Here's the drawing with two shaded views (mm, measured from the low corner). I have some questions. A direction names the side the tool comes from. Coordinates: 2 decimals unless noted, no trailing zeros. Loops run counter-clockwise (first coordinate to the right, second up) from the corner with the lowest first, then second, coordinate; pieces in that order, holes last. Notation, with made-up numbers: M 60,-10 L 84,-10 A33 cw 84,26 Z; hole C 78.25,58.5 d4. An arc over 180 degrees is marked long. Return JSON: item names as keys, results as strings. Group by question number.
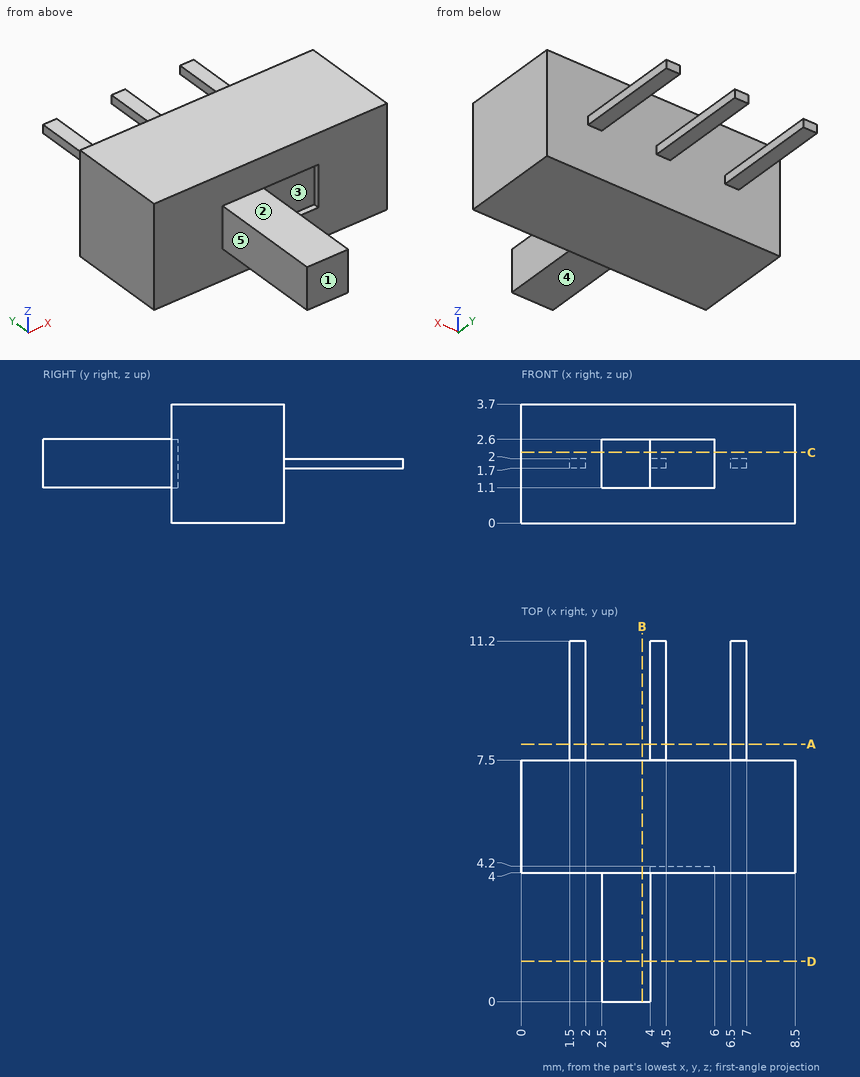
1) If we mould it in two halves opening along Z, with no side actions, what happens to the marked faces 3, 4 and 5? For each: +Z half, -Z half, draft (parallel to the pull), parting line (faces both ways), or undercut.
2) Suppose I cut it at D-D, the plane y = 1.25. List the corners of the cut face in (x, z) for me.
3) Suppose I cut it at B-B, the plane x = 3.75. List the corners of the cut face in (y, z) for me, then the cut area to 4 significant figures.
4) Suppose I cut it at A-A, the plane y = 8. List the corners of the cut face in (x, z) for me.
5) Suppose I cut it at C-C, the plane z = 2.2. List the corners of the cut face in (x, y) for me.
6) If I drill on line 1 (Y direction, x = 8.25, z = 0.9); line 2 (Y direction, x = 5, z = 1.45); line 3 (X direction, y = 3.5, z = 1.7), over which ranges is the centre line in solid material (lowest first)? Write a range as from..to.
7) For pin 1 (1.1 mm diameter, centred on x = 5.5, z = 2, fed in from +Y); pin 2 (0.8 mm diameter, centred on x = 3.5, y = 1.5, fed in from +Z), each with a flat end and sliding along its axis, tell me the tip position at first contact or that it passes through.
8) For the marked faces 1 and 2, which set-ups out of +Z, -Z, +X, -X, +Y, -Y let a thin tool reach every point of the face, with its end or its side?
Returned:
{
 "1": {"face 3": "undercut", "face 4": "-Z half", "face 5": "draft"},
 "2": {"outline": "M 2.5,1.1 L 4,1.1 L 4,2.6 L 2.5,2.6 Z"},
 "3": {"outline": "M 0,1.1 L 4,1.1 L 4,0 L 7.5,0 L 7.5,3.7 L 4,3.7 L 4,2.6 L 0,2.6 Z", "area": "18.95 mm²"},
 "4": {"outline": "M 1.5,1.7 L 2,1.7 L 2,2 L 1.5,2 Z; M 4,1.7 L 4.5,1.7 L 4.5,2 L 4,2 Z; M 6.5,1.7 L 7,1.7 L 7,2 L 6.5,2 Z"},
 "5": {"outline": "M 0,4 L 2.5,4 L 2.5,0 L 4,0 L 4,4.2 L 6,4.2 L 6,4 L 8.5,4 L 8.5,7.5 L 0,7.5 Z"},
 "6": {"line 1": "y = 4..7.5", "line 2": "y = 4.2..7.5", "line 3": "x = 2.5..4"},
 "7": {"pin 1": "stops at y = 7.5", "pin 2": "stops at z = 2.6"},
 "8": {"face 1": "+Z, -Z, +X, -X, -Y", "face 2": "+Z, +X, -X, -Y"}
}
